CAD build for the part. Positions are in the model's coordinates, mm. A direction names the side the tool comes from. Round coordinates to 2 decimals unless told otherwise and drop trailing zeros. Order: outer loops, then holes, each group sorted by start corner. A loop starts at its lowest first (then second) coordinate and runs counter-clockwise, first axis right, second up. Notation, with made-up numbers: M 19,54.25 L 49,54.25 A8 cw 49,67.25 Z; hole C 28.5,66.5 d8. An arc over 180 degrees is marked long. Put each result on its own line as item: value.
```python
from build123d import *

# Parameters (mm, degrees)
SKETCH1_W                             = 82.55
SKETCH1_H                             = 69.85
BOSS_EXTRUDE1_DEPTH                   = 7.9375
SKETCH2_W                             = 82.55
SKETCH2_H                             = 69.85
BOSS_EXTRUDE2_DEPTH                   = 3.175
F_3_8_16_TAPPED_HOLE1_D               = 7.9375
F_3_8_16_TAPPED_HOLE1_DEPTH           = 9.525
F_3_8_16_TAPPED_HOLE1_TIP             = 2.384665582
DRAFT1_ANGLE                          = 5
SKETCH3_W                             = 12.7
SKETCH3_H                             = 69.85
BOSS_EXTRUDE3_DEPTH                   = 7.9375
SKETCH4_W                             = 13.267261336
SKETCH4_H                             = 69.85
SKETCH4_W_2                           = 17.684109612
WEAR_PADS_DEPTH                       = 1.5875
F_10_24_TAPPED_HOLE1_D                = 3.7973
F_10_24_TAPPED_HOLE1_DEPTH            = 12.7
F_1_4_0_25_DIAMETER_HOLE1_D           = 6.35
F_1_4_0_25_DIAMETER_HOLE1_DEPTH       = 8.89
F_1_4_0_25_DIAMETER_HOLE1_CSINK_D     = 7.62
F_1_4_0_25_DIAMETER_HOLE1_CSINK_ANGLE = 90
F_1_4_0_25_DIAMETER_HOLE1_TIP         = 1.907732465


with BuildPart() as part:
    # Sketch1 → Boss-Extrude1 (new body)
    with BuildSketch(Plane(origin=(0, 0, 0), x_dir=(1, 0, 0), z_dir=(0, 1, 0))):
        Rectangle(SKETCH1_W, SKETCH1_H)
    extrude(amount=BOSS_EXTRUDE1_DEPTH)

    # Sketch2 → Boss-Extrude2 (add)
    with BuildSketch(Plane(origin=(0, 7.9375, 0), x_dir=(1, 0, 0), z_dir=(0, 1, 0))):
        Rectangle(SKETCH2_W, SKETCH2_H)
    extrude(amount=BOSS_EXTRUDE2_DEPTH)

    # 3/8-16 Tapped Hole1
    with Locations(Plane(origin=(0, 11.1125, 0), x_dir=(1, 0, 0), z_dir=(0, 1, 0))):
        with Locations((-25.4, -19.05), (25.4, -19.05)):
            Hole(F_3_8_16_TAPPED_HOLE1_D / 2, depth=F_3_8_16_TAPPED_HOLE1_DEPTH)
            with Locations((0, 0, -(F_3_8_16_TAPPED_HOLE1_DEPTH + F_3_8_16_TAPPED_HOLE1_TIP / 2))):  # 118° drill point
                Cone(0, F_3_8_16_TAPPED_HOLE1_D / 2, F_3_8_16_TAPPED_HOLE1_TIP, mode=Mode.SUBTRACT)

    # Draft1
    draft1_faces = [part.faces().sort_by_distance(p)[0] for p in [
        (0, 5.55625, -34.925),
        (-41.275, 5.55625, 0),
        (0, 5.55625, 34.925),
        (41.275, 5.55625, 0),
    ]]
    draft(draft1_faces, Plane.ZX, DRAFT1_ANGLE)

    # Sketch3 → Boss-Extrude3 (add)
    with BuildSketch(Plane.XZ):
        with Locations((34.925, 0)):
            Rectangle(SKETCH3_W, SKETCH3_H)
        with Locations((-34.925, 0)):
            Rectangle(SKETCH3_W, SKETCH3_H)
    extrude(amount=BOSS_EXTRUDE3_DEPTH)

    # Sketch4 → Wear Pads (add)
    with BuildSketch(Plane.XZ):
        with Locations((-21.941369332, 0)):
            Rectangle(SKETCH4_W, SKETCH4_H)
        with Locations((19.732945194, 0)):
            Rectangle(SKETCH4_W_2, SKETCH4_H)
    extrude(amount=WEAR_PADS_DEPTH)

    # #10-24 Tapped Hole1
    with Locations(Plane(origin=(41.275, 0, 0), x_dir=(0, 0, -1), z_dir=(1, 0, 0))):
        with Locations((-25.4, -5.151627132), (25.4, -5.151627132), (0, -5.151627132)):
            Hole(F_10_24_TAPPED_HOLE1_D / 2, depth=F_10_24_TAPPED_HOLE1_DEPTH)

    # 1/4 (0.25) Diameter Hole1
    with Locations(Plane(origin=(0, 11.1125, 0), x_dir=(1, 0, 0), z_dir=(0, 1, 0))):
        with Locations((-15.817703685, 27.018390392), (23.931088267, 27.018390392)):
            CounterSinkHole(F_1_4_0_25_DIAMETER_HOLE1_D / 2, F_1_4_0_25_DIAMETER_HOLE1_CSINK_D / 2, depth=F_1_4_0_25_DIAMETER_HOLE1_DEPTH, counter_sink_angle=F_1_4_0_25_DIAMETER_HOLE1_CSINK_ANGLE)
            with Locations((0, 0, -(F_1_4_0_25_DIAMETER_HOLE1_DEPTH + F_1_4_0_25_DIAMETER_HOLE1_TIP / 2))):  # 118° drill point
                Cone(0, F_1_4_0_25_DIAMETER_HOLE1_D / 2, F_1_4_0_25_DIAMETER_HOLE1_TIP, mode=Mode.SUBTRACT)


solid = part.part
```
Item 1: Band-saw the part on B-B on x = -25.4. Give the cut face in (y, z) (1 decimal).
Answers below:
outline: M -1.6,-34.9 L 0,-34.9 L 11.1,-34 L 11.1,15.1 L 1.6,15.1 L 0,17.7 L 0,20.4 L 1.6,23 L 11.1,23 L 11.1,34 L 0,34.9 L -1.6,34.9 Z
Item 2: Band-saw the part on C-C on y = 5.5. State how many separate pieces and enclosed holes the cut face has, and give its area (3 significant figures).
Answers below:
separate pieces: 1
enclosed holes: 4
area: 5,460 mm²
Item 3: Pin check, flat tips, straight feed: P1, Ø0.8, axis at x = -26, z = 19.5, coming from the +Y side; P2, Ø5, axis at x = -25.4, z = 19.05, coming from the -Y side; P3, Ø4, axis at x = -0.5, z = -8.5, coming from the -Y side. Stop position of each tip, or through.
Answers below:
P1: y = 0
P2: y = -1.59
P3: y = 0
Item 4: Tool access for faces 4 (the cylindrical face through (34.836, -5.068, 23.503)), 5 (the cylindrical face through (28.325, 6.283, 16.368)), 6 (the flat face through (-2, 0, 0)): list every direction of +Z, -Z, +X, -X, +Y, -Y with a clear straight run to the whole face (end or side of a thin tool).
Answers below:
face 4: +X
face 5: +Y
face 6: +Z, -Z, -Y
Item 5: Probe line 1 along X through (y, z) = (-3.5, 15) (3 decimals); line 2 along X through (y, z) = (-1, 12) (3 decimals); line 3 along Y through (x, z) = (34.75, -25.4). List the from-to ranges inside material, lowest first. Write a range as [from, to].
Answers below:
line 1: [-41.275, -28.575], [28.575, 41.275]
line 2: [-41.275, -15.308], [10.891, 41.275]
line 3: [-7.94, -7.05], [-3.25, 11.11]
Item 6: Band-saw the part on A-A on z = 0. Give the cut face in (x, y) (1 decimal).
Answers below:
outline: M -41.3,-7.9 L -28.6,-7.9 L -28.6,-1.6 L -15.3,-1.6 L -15.3,0 L 10.9,0 L 10.9,-1.6 L 28.6,-1.6 L 28.6,-3.3 L 41.3,-3.3 L 41.3,0 L 40.3,11.1 L -40.3,11.1 L -41.3,0 Z; M 28.6,-7.9 L 41.3,-7.9 L 41.3,-7.1 L 28.6,-7.1 Z
Item 7: Mould opens along Z. For faces 1 (the flat face through (-34, -3, -34.925)), 2 (the conical face through (-25.72, 0.1, 20.51)), 3 (the flat face through (-22, -1.588, 0)) say: pulls with the +Z half, pulls with the -Z half, needs draft (parallel to the pull), parting line crosses it, or undercut.
Answers below:
face 1: pulls with the -Z half
face 2: undercut
face 3: needs draft
Item 8: Band-saw the part on D-D on z = -14.5. Give the cut face in (x, y) (1 decimal).
Answers below:
outline: M -41.3,-7.9 L -28.6,-7.9 L -28.6,-1.6 L -15.3,-1.6 L -15.3,0 L 10.9,0 L 10.9,-1.6 L 28.6,-1.6 L 28.6,-7.9 L 41.3,-7.9 L 41.3,0 L 40.3,11.1 L -40.3,11.1 L -41.3,0 Z
